Model file for the job. Use its own axes, mm. Round coordinates to 2 decimals unless told otherwise and drop trailing zeros. Order: outer loops, then holes, each group sorted by start corner. A loop starts at its lowest first (then second) coordinate and runs counter-clockwise, first axis right, second up. Notation, with made-up numbers: (-2.5, -4.5) - (34.5, -4.5) arc R19 cw to (34.5, -0.5) - close; hole circle Ø9 at (-21, 33). An arc over 180 degrees is marked (long way). Use one line per item in the form item = value.
from build123d import *

# Parameters (mm, degrees)
SKETCH1_W           = 100
SKETCH1_H           = 300
BOSS_EXTRUDE1_DEPTH = 2
SKETCH2_R           = 1
CUT_EXTRUDE1_DEPTH  = 10
SKETCH3_R           = 17.5
CUT_EXTRUDE2_DEPTH  = 10
SKETCH5_R           = 1
CUT_EXTRUDE3_DEPTH  = 10


with BuildPart() as part:
    # Sketch1 → Boss-Extrude1 (new body)
    with BuildSketch(Plane.XY):
        Rectangle(SKETCH1_W, SKETCH1_H)
    extrude(amount=BOSS_EXTRUDE1_DEPTH)

    # Sketch2 → Cut-Extrude1 (cut)
    with BuildSketch(Plane.XY.offset(2)):
        with Locations((-39, 122)):
            Circle(SKETCH2_R)
        with Locations((-39, 77)):
            Circle(SKETCH2_R)
        with Locations((39, 122)):
            Circle(SKETCH2_R)
        with Locations((39, 77)):
            Circle(SKETCH2_R)
        with Locations((-39, 21)):
            Circle(SKETCH2_R)
        with Locations((-39, -24)):
            Circle(SKETCH2_R)
        with Locations((39, 21)):
            Circle(SKETCH2_R)
        with Locations((39, -24)):
            Circle(SKETCH2_R)
        with Locations((-39, -80)):
            Circle(SKETCH2_R)
        with Locations((-39, -125)):
            Circle(SKETCH2_R)
        with Locations((39, -80)):
            Circle(SKETCH2_R)
        with Locations((39, -125)):
            Circle(SKETCH2_R)
        with Locations((16.5, -146.5)):
            Circle(SKETCH2_R)
        with Locations((-16.5, -146.5)):
            Circle(SKETCH2_R)
        with Locations((-16.5, 146.5)):
            Circle(SKETCH2_R)
        with Locations((16.5, 146.5)):
            Circle(SKETCH2_R)
    extrude(amount=-CUT_EXTRUDE1_DEPTH, mode=Mode.SUBTRACT)

    # Sketch3 → Cut-Extrude2 (cut)
    with BuildSketch(Plane(origin=(0, 0, 0), x_dir=(-1, 0, 0), z_dir=(0, 0, -1))):
        with Locations((0, 91)):
            Circle(SKETCH3_R)
    extrude(amount=-CUT_EXTRUDE2_DEPTH, mode=Mode.SUBTRACT)

    # Sketch5 → Cut-Extrude3 (cut)
    with BuildSketch(Plane.XY.offset(2)):
        with Locations((-16.5, 47.5)):
            Circle(SKETCH5_R)
        with Locations((16.5, 47.5)):
            Circle(SKETCH5_R)
        with Locations((-16.5, -47.5)):
            Circle(SKETCH5_R)
        with Locations((16.5, -47.5)):
            Circle(SKETCH5_R)
    extrude(amount=-CUT_EXTRUDE3_DEPTH, mode=Mode.SUBTRACT)


solid = part.part
(1) Slice it at C-C on z = 0.35. Count the separate pieces of the cut face and the enclosed holes in it, then the cut area to 3 significant figures.
Report:
separate_pieces = 1
enclosed_holes = 21
area = 29,000 mm2
(2) Slice it at B-B on x = 0. Give the cut face in (y, z).
Report:
outline = (-150, 0) - (73.5, 0) - (73.5, 2) - (-150, 2) - close; (108.5, 0) - (150, 0) - (150, 2) - (108.5, 2) - close
(3) Pull direction X, two halves, no side cores. Call faces 1 (the face through (-1, 2, 0)), 2 (the face through (3.794, 73.916, 0.986)): released by +X, released by -X, zero draft, split by the parting line, or undercut.
Report:
face_1 = zero draft
face_2 = undercut
(4) Probe probe 1 along X at (y, z) = (146.5, 0.65); probe 2 along X at (y, z) = (-125, 1.4); probe 3 along X at (y, z) = (77, 0.9). List the from-to ranges inside material, lowest first. Write a range as [from, to].
Report:
probe_1 = [-50, -17.5], [-15.5, 15.5], [17.5, 50]
probe_2 = [-50, -40], [-38, 38], [40, 50]
probe_3 = [-50, -40], [-38, -10.5], [10.5, 38], [40, 50]
(5) Slice it at A-A on y = 91. Give the cut face in (x, z).
Report:
outline = (-50, 0) - (-17.5, 0) - (-17.5, 2) - (-50, 2) - close; (17.5, 0) - (50, 0) - (50, 2) - (17.5, 2) - close
(6) Pin check, flat tip, straight feed: pin 1 (1.2 mm diameter, centred on x = -16.5, y = 47.5, fed in from +Z). Stop position of the tip, or through.
Report:
pin_1 = through
